Can you work these out from the model? Positions are in its coordinate system, mm. Face numbers are marked on the shaded views. A direction names the side the tool comes from. Coordinates: 2 decimals unless noted, no trailing zeros. Loops run counter-clockwise (first coordinate to the right, second up) from the corner with the lowest first, then second, coordinate; pieces in that order, holes last.
```python
from build123d import *

# Parameters (mm, degrees)
SKETCH1_W                                       = 152.4
SKETCH1_H                                       = 157.48
BOSS_EXTRUDE1_DEPTH                             = 9.525
SKETCH16_W                                      = 152.4
SKETCH16_H                                      = 9.525
BOSS_EXTRUDE2_DEPTH                             = 2.54
M100_CLEARANCE_HOLE1_D                          = 106.553
M100_CLEARANCE_HOLE1_DEPTH                      = 1.3462
SKETCH4_W                                       = 63.5
SKETCH4_H                                       = 19.05
SKETCH5_W                                       = 50.6095
SKETCH5_H                                       = 1.3462
CBORE_FOR_10_SOCKET_HEAD_CAP_SCREW1_D           = 5.1054
CBORE_FOR_10_SOCKET_HEAD_CAP_SCREW1_CBORE_D     = 9.525
CBORE_FOR_10_SOCKET_HEAD_CAP_SCREW1_CBORE_DEPTH = 4.826
F_10_24_TAPPED_HOLE1_D                          = 3.7973
F_10_24_TAPPED_HOLE1_DEPTH                      = 8.89
F_10_24_TAPPED_HOLE1_TIP                        = 1.140824014
M90_CLEARANCE_HOLE1_D                           = 95.25
M90_CLEARANCE_HOLE1_DEPTH                       = 12.7
M36_CLEARANCE_HOLE1_D                           = 41.148
M36_CLEARANCE_HOLE1_DEPTH                       = 15.875
F_10_24_TAPPED_HOLE2_D                          = 3.7973
F_10_24_TAPPED_HOLE2_DEPTH                      = 7.74954
F_10_24_TAPPED_HOLE2_TIP                        = 1.140824014


with BuildPart() as part:
    # Sketch1 → Boss-Extrude1 (new body)
    with BuildSketch(Plane(origin=(0, 0, 0), x_dir=(-1, 0, 0), z_dir=(0, 0, -1))):
        with Locations((0, -2.54)):
            Rectangle(SKETCH1_W, SKETCH1_H)
    extrude(amount=-BOSS_EXTRUDE1_DEPTH)

    # Sketch16 → Boss-Extrude2 (add)
    with BuildSketch(Plane(origin=(0, 76.2, 0), x_dir=(1, 0, 0), z_dir=(0, 1, 0))):
        with Locations((0, -4.7625)):
            Rectangle(SKETCH16_W, SKETCH16_H)
    extrude(amount=BOSS_EXTRUDE2_DEPTH)

    # M100 Clearance Hole1
    with Locations(Plane.XY.offset(9.525)):
        with Locations((0, 0)):
            Hole(M100_CLEARANCE_HOLE1_D / 2, depth=M100_CLEARANCE_HOLE1_DEPTH)

    # Sketch4 → Revolve1 (revolve)
    with BuildSketch(Plane(origin=(0, 0, 0), x_dir=(1, 0, 0), z_dir=(0, 1, 0))):
        with Locations((31.75, 9.525)):
            Rectangle(SKETCH4_W, SKETCH4_H)
    revolve(axis=Axis((0, 0, -19.05), (0, 0, 1)))

    # Sketch5 → Revolve2 (revolve)
    with BuildSketch(Plane(origin=(0, 0, 0), x_dir=(1, 0, 0), z_dir=(0, 1, 0))):
        with Locations((25.30475, -8.8519)):
            Rectangle(SKETCH5_W, SKETCH5_H)
    revolve(axis=Axis((0, 0, 8.1788), (0, 0, 1)))

    # CBORE for #10 Socket Head Cap Screw1 (through all)
    with Locations(Plane(origin=(0, 0, 0), x_dir=(-1, 0, 0), z_dir=(0, 0, -1))):
        with Locations((71.12, 38.1), (71.12, -38.1), (-71.12, 38.1), (-71.12, -38.1), (0, 72.009), (0, -72.009), (71.12, 0), (-71.12, 0)):
            CounterBoreHole(CBORE_FOR_10_SOCKET_HEAD_CAP_SCREW1_D / 2, CBORE_FOR_10_SOCKET_HEAD_CAP_SCREW1_CBORE_D / 2, CBORE_FOR_10_SOCKET_HEAD_CAP_SCREW1_CBORE_DEPTH)

    # #10-24 Tapped Hole1
    with Locations(Plane(origin=(0, 0, -19.05), x_dir=(-1, 0, 0), z_dir=(0, 0, -1))):
        with Locations((17.311395212, 15.494), (17.311395212, -15.494), (-9.525, -30.988), (-36.361395212, -15.494), (-36.361395212, 15.494), (-9.525, 30.988)):
            Hole(F_10_24_TAPPED_HOLE1_D / 2, depth=F_10_24_TAPPED_HOLE1_DEPTH)
            with Locations((0, 0, -(F_10_24_TAPPED_HOLE1_DEPTH + F_10_24_TAPPED_HOLE1_TIP / 2))):  # 118° drill point
                Cone(0, F_10_24_TAPPED_HOLE1_D / 2, F_10_24_TAPPED_HOLE1_TIP, mode=Mode.SUBTRACT)

    # M90 Clearance Hole1
    with Locations(Plane.XY.offset(9.525)):
        with Locations((0, 0)):
            Hole(M90_CLEARANCE_HOLE1_D / 2, depth=M90_CLEARANCE_HOLE1_DEPTH)

    # M36 Clearance Hole1
    with Locations(Plane.XY.offset(-3.175)):
        with Locations((9.525, 0)):
            Hole(M36_CLEARANCE_HOLE1_D / 2, depth=M36_CLEARANCE_HOLE1_DEPTH)

    # #10-24 Tapped Hole2
    with Locations(Plane.XY.offset(-3.175)):
        with Locations((14.2875, -24.746675913), (-28.575, 0), (14.2875, 24.746675913)):
            Hole(F_10_24_TAPPED_HOLE2_D / 2, depth=F_10_24_TAPPED_HOLE2_DEPTH)
            with Locations((0, 0, -(F_10_24_TAPPED_HOLE2_DEPTH + F_10_24_TAPPED_HOLE2_TIP / 2))):  # 118° drill point
                Cone(0, F_10_24_TAPPED_HOLE2_D / 2, F_10_24_TAPPED_HOLE2_TIP, mode=Mode.SUBTRACT)


solid = part.part
```
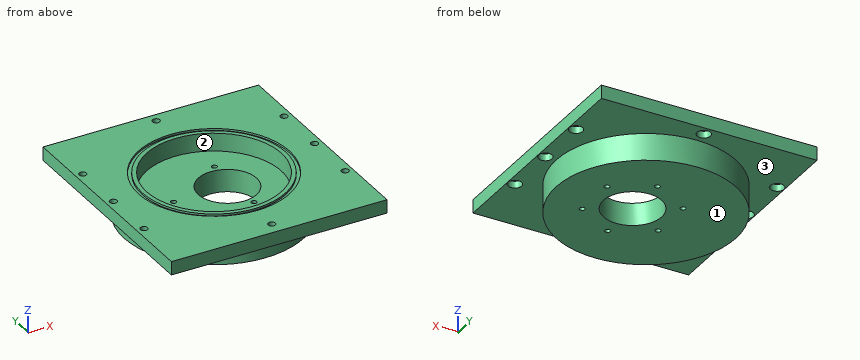
Item 1: On a 3-axis mill with a long thin cutter (end or side, diameter ignored), from which of +Z, -Z, +X, -X, +Y, -Y can I reach the whole of each face in a straight line? I mean the marked faces 1, 2 and 3. Say none if no direction works.
Results are:
face 1: -Z, +X, -X, +Y, -Y
face 2: +Z
face 3: -Z
Item 2: I'm going to push flat-ended pins straight in: P1, Ø7.5, axis at x = -71.12, y = 38.1, coming from the -Z side; P2, Ø7.5, axis at x = 0, y = 74.5, coming from the -Z side; P3, Ø6, axis at x = 8, z = -11, coming from the -Y side; P4, Ø3, axis at x = -71.12, y = -38.1, coming from the +Z side. Where does each tip first touch, or does it pass through?
Results are:
P1: stops at z = 4.83
P2: stops at z = 0
P3: stops at y = -63.3
P4: passes through
Item 3: I need wall thicknesses on line 1 along Y through (x, z) = (71.12, 2.9); line 2 along Y through (x, z) = (-71.12, 7.6); line 3 along X through (y, z) = (-40, 1). Which ranges of each line are inside material? Lowest first, please.
Results are:
line 1: y = -81.28 to -42.86, -33.34 to -4.76, 4.76 to 33.34, 42.86 to 78.74
line 2: y = -81.28 to -40.65, -35.55 to -2.55, 2.55 to 35.55, 40.65 to 78.74
line 3: x = -76.2 to -75.49, -66.75 to -25.85, 25.85 to 66.75, 75.49 to 76.2
Item 4: Suppose I cut it at A-A, the plane x = -71.12. Please give me the cut outline in (y, z) (1 decimal).
Results are:
outline: (-81.3, 0) - (-42.9, 0) - (-42.9, 4.8) - (-40.7, 4.8) - (-40.7, 9.5) - (-81.3, 9.5) - close; (-35.5, 4.8) - (-33.3, 4.8) - (-33.3, 0) - (-4.8, 0) - (-4.8, 4.8) - (-2.6, 4.8) - (-2.6, 9.5) - (-35.5, 9.5) - close; (2.6, 4.8) - (4.8, 4.8) - (4.8, 0) - (33.3, 0) - (33.3, 4.8) - (35.5, 4.8) - (35.5, 9.5) - (2.6, 9.5) - close; (40.7, 4.8) - (42.9, 4.8) - (42.9, 0) - (78.7, 0) - (78.7, 9.5) - (40.7, 9.5) - close
Item 5: Suppose I cut it at C-C, the plane z = 2.5. Count the separate pieces of the cut face and the enclosed holes in it, plus the area to 3 significant figures.
Results are:
separate pieces: 1
enclosed holes: 9
area: 16,700 mm2
Item 6: Suppose I cut it at D-D, the plane x = -35.5. Please give me the cut outline in (y, z) (3 decimals).
Results are:
outline: (-81.28, 0) - (-52.65, 0) - (-52.65, -19.05) - (52.65, -19.05) - (52.65, 0) - (78.74, 0) - (78.74, 9.525) - (39.726, 9.525) - (39.726, 8.179) - (36.07, 8.179) - (36.07, 9.525) - (31.747, 9.525) - (31.747, -3.175) - (-31.747, -3.175) - (-31.747, 9.525) - (-36.07, 9.525) - (-36.07, 8.179) - (-39.726, 8.179) - (-39.726, 9.525) - (-81.28, 9.525) - close
Item 7: Suppose I cut it at B-B, the plane z = -17. Please give me the cut outline in (x, y) (3 decimals), plus the area to 3 significant figures.
Results are:
outline: circle Ø127 at (0, 0); hole circle Ø3.797 at (-17.311, -15.494); hole circle Ø3.797 at (-17.311, 15.494); hole circle Ø41.148 at (9.525, 0); hole circle Ø3.797 at (9.525, -30.988); hole circle Ø3.797 at (9.525, 30.988); hole circle Ø3.797 at (36.361, -15.494); hole circle Ø3.797 at (36.361, 15.494)
area: 11,300 mm2
